The listing builds one solid part. Answer for the finished solid, in the listing's coordinates (mm). A direction names the side the tool comes from. Round coordinates to 2 decimals unless told otherwise and drop trailing zeros. Loops run counter-clockwise (first coordinate to the right, second up) from the corner with the lowest first, then second, coordinate; pieces in that order, holes last. Notation, with made-up numbers: M 86.5,68 L 99.5,68 A24 ccw 99.5,81 Z; hole C 50,12 d4. An arc over 180 degrees is marked long. Answer as a JSON object with one key per item and string values.
Autodesk Inventor part; units mm, degrees
ref_plane "YZ Plane" through (0, 0, 0) normal (1, 0, 0) x (0, 1, 0)
ref_plane "XZ Plane" through (0, 0, 0) normal (0, 1, 0) x (-1, 0, 0)
ref_plane "XY Plane" through (0, 0, 0) normal (0, 0, 1) x (1, 0, 0)
sketch "Sketch1" plane through (0, 0, 0) normal (0, 1, 0) x (-1, 0, 0)
  line L0 (46.923, -68.9252) -> (29.323, -68.9252)
  line L1 (29.323, -68.9252) -> (29.323, -48.7252)
  line L2 (29.323, -48.7252) -> (46.923, -48.7252)
  line L3 (46.923, -48.7252) -> (46.923, -68.9252)
  point P0 (0, 0)
  dimension "d0" = 17.6
  dimension "d1" = 20.2
extrude "Extrusion1" add sketch "Sketch1" along normal blind 8.5
sketch "Sketch2" plane through (-29.323, 0, -48.7252) normal (1, 0, 0) x (0, 0, -1)
  line L0 (0, 0) -> (20.2, 0)
  line L1 (20.2, 0) -> (20.2, 8.5)
  line L2 (0, 8.5) -> (20.2, 8.5)
  line L3 (0, 0) -> (0, 8.5)
  line L4 (20.2, 0) -> (20.2, 8.5)
  line L5 (20.2, 4.25) -> (0, 4.25)
  line L6 (0, 0) -> (0, 8.5)
  circle A0 centre (15.1699, 4.25) radius 2
  point P0 (-48.7252, 0)
  dimension "d4" = 4
extrude "Extrusion2" add sketch "Sketch2" along normal blind 3 contours A0 L5 | L5 A0
properties part number "servo_cos"
Item 1: Flat-ended cylindrical pins translate along their axes: P1, Ø2.5, axis at y = 6, z = -61, coming from the +X side; P2, Ø3, axis at x = -30, z = -62.5, coming from the -Y side. Find the tip coordinate at first contact, or state that the pin passes through.
Values follow:
{"P1": "x = -29.32", "P2": "y = 0"}
Item 2: The part is cut by section B-B (z = -58.75). Give the vertices of the cut face in (x, y), then the cut area to 3 significant figures.
Values follow:
{"outline": "M -46.92,0 L -29.32,0 L -29.32,8.5 L -46.92,8.5 Z", "area": "150 mm^2"}
Item 3: The part is cut by section C-C (z = -64.5). Give the vertices of the cut face in (x, y), then the cut area to 3 significant figures.
Values follow:
{"outline": "M -46.92,0 L -29.32,0 L -29.32,2.34 L -26.32,2.34 L -26.32,6.16 L -29.32,6.16 L -29.32,8.5 L -46.92,8.5 Z", "area": "161 mm^2"}
Item 4: Straight lines are drawn through the part: line 1 (X direction, y = 7, z = -50.75); line 2 (Z direction, x = -27.5, y = 3); line 3 (Z direction, x = -27.5, y = 5). For each, find the intervals that lie inside material, in ascending order.
Values follow:
{"line 1": "-46.92 to -29.32", "line 2": "-65.46 to -62.33", "line 3": "-65.75 to -62.04"}
Item 5: Which of the six approach directions +Z, -Z, +X, -X, +Y, -Y give full straight-line access (tool end or side, diameter ignored) to faces 1 (the face through (-46.923, 4, -59)), 2 (the face through (-27.844, 4.162, -61.897))?
Values follow:
{"face 1": "+Z, -Z, -X, +Y, -Y", "face 2": "+X"}
Item 6: The part is cut by section A-A (y = 4.25). Give the vertices of the cut face in (x, z).
Values follow:
{"outline": "M -46.92,-68.93 L -29.32,-68.93 L -29.32,-65.9 L -26.32,-65.9 L -26.32,-61.9 L -29.32,-61.9 L -29.32,-48.73 L -46.92,-48.73 Z"}
Item 7: The part is cut by section D-D (y = 7.75). Give the vertices of the cut face in (x, z), then the cut area to 3 significant figures.
Values follow:
{"outline": "M -46.92,-68.93 L -29.32,-68.93 L -29.32,-48.73 L -46.92,-48.73 Z", "area": "356 mm^2"}
